The listing builds one solid part. Answer for the finished solid, in the listing's coordinates (mm). A direction names the side the tool comes from. Round coordinates to 2 decimals unless told otherwise and drop trailing zeros. Order: outer loops, then holes, each group sorted by start corner. A loop starts at its lowest first (then second) coordinate and runs counter-clockwise, first axis right, second up. Notation, with made-up numbers: (59.5, 59.25) - (68.5, 59.25) arc R20 cw to (68.5, 78.25) - close; hole circle Ø1 at (59, 48.25). An arc over 180 degrees is marked (long way). Use CSV: the item, a comma, the result in double quotes. Start each with the question number.
Item 1: Determine the mould class of faces 1 (the flat face through (-11.47, -24.65, -11.16)), 2 (the flat face through (-7.669, -24.65, -7.887)), 3 (the flat face through (-8, 0, -8)) for opening direction Z: +Z half, -Z half, draft (parallel to the pull), parting line (faces both ways), or undercut.
Item 2: Find section C-C, the plane z = 5. Give the vertices of the cut face in (x, y).
Item 3: Flat-ended cylindrical pins translate along their axes: P1, Ø1.5, axis at y = -30.5, z = -12, coming from the +X side; P2, Ø12, axis at y = -9.5, z = -18, coming from the +X side; P3, Ø1.5, axis at y = -24.5, z = -7.5, coming from the -X side. Find the tip coordinate at first contact, or state that the pin passes through.
Item 4: Find section B-B, the plane x = 5.5. Give the vertices of the cut face in (y, z), plus the area to 3 significant figures.
Item 5: Find section D-D, the plane z = 18. Give the vertices of the cut face in (x, y), plus the area to 3 significant figures.
Item 6: For faces 4 (the flat face through (-8, -50, -8)), 5 (the flat face through (7.887, -24.65, -7.669)), determine the directions among +Z, -Z, +X, -X, +Y, -Y from which every point of the face is accessible in a straight line to the end or side of a thin tool.
Item 7: Find section A-A, the plane y = -44. Give the vertices of the cut face in (x, z).
Item 8: Straight lines are drawn through the part: line 1 along Z through (x, y) = (14.5, -19.5); line 2 along X through (y, z) = (-34, 3); line 3 along X through (y, z) = (-36, -10). For each, find the intervals that lie inside material, in ascending order. Write a range as [from, to].
```python
from build123d import *

# Parameters (mm, degrees)
F1_DEPTH = 50


with BuildPart() as f1:
    # F0 (on Front) → F1 (new body)
    with BuildSketch(Plane.XZ):
        Polygon((0, 22.627417), (-22.627417, 0), (0, -22.627417), (22.627417, 0), align=None)
        Polygon((-15.556349, 0), (0, 15.556349), (15.556349, 0), (0, -15.556349), align=None, mode=Mode.SUBTRACT)
    extrude(amount=F1_DEPTH)


solid = f1.part
```
Worked out:
1,face 1,"-Z half"
1,face 2,"undercut"
1,face 3,"draft"
2,outline,"(-17.63, -50) - (-10.56, -50) - (-10.56, 0) - (-17.63, 0) - close; (10.56, -50) - (17.63, -50) - (17.63, 0) - (10.56, 0) - close"
3,P1,"stops at x = 11.38"
3,P2,"stops at x = 10.63"
3,P3,"stops at x = -15.88"
4,outline,"(-50, -17.13) - (0, -17.13) - (0, -10.06) - (-50, -10.06) - close; (-50, 10.06) - (0, 10.06) - (0, 17.13) - (-50, 17.13) - close"
4,area,"707 mm²"
5,outline,"(-4.63, -50) - (4.63, -50) - (4.63, 0) - (-4.63, 0) - close"
5,area,"463 mm²"
6,face 4,"+Z, -Z, +X, -X, -Y"
6,face 5,"+Y, -Y"
7,outline,"(-22.63, 0) - (0, -22.63) - (22.63, 0) - (0, 22.63) - close; hole (-15.56, 0) - (0, -15.56) - (15.56, 0) - (0, 15.56) - close"
8,line 1,"z = [-8.13, -1.06], [1.06, 8.13]"
8,line 2,"x = [-19.63, -12.56], [12.56, 19.63]"
8,line 3,"x = [-12.63, -5.56], [5.56, 12.63]"
